The listing builds one solid part. Answer for the finished solid, in the listing's coordinates (mm). Face numbers are marked on the shaded views. A direction names the side the tool comes from. Give positions to 0.01 mm unless a question says otherwise; leave off trailing zeros. Order: outer loops, then holes, each group sorted by start corner. A loop starts at its lowest first (then second) coordinate and runs counter-clockwise, first axis right, second up. Notation, with made-up numbers: (76.25, 30) - (123.25, 30) arc R18 cw to (123.25, 42) - close; hole circle Ø3 at (-30.75, -34). An arc over 180 degrees is marked (long way). Answer as CSV lines item,"result". Start each with the question number.
1. Determine the mould class of the marked faces 1, 2 and 3 for opening direction Y: +Y half, -Y half, draft (parallel to the pull), parting line (faces both ways), or undercut.
2. Which of the six approach directions +Z, -Z, +X, -X, +Y, -Y give full straight-line access (tool end or side, diameter ignored) to the marked faces 4 and 5?
3. Section D-D on x = 19.5 is taken. Give the vertices of the cut face in (y, z).
4. Consider line 1 along Y through (x, z) = (0, 4.5); line 2 along Y through (x, z) = (0, 0.85); line 3 along Z through (x, y) = (-22.5, 13.5). Determine where each line is inside the solid, lowest interval first. Write a range as [from, to].
5. Section C-C on z = 1 is taken. Give the vertices of the cut face in (x, y), and give its area (3 significant figures).
6. Section A-A on y = 0 is taken. Give the vertices of the cut face in (x, z), and give its area (3 significant figures).
7. Flat-ended cylindrical pins translate along their axes: pin 1 (1.5 mm diameter, centred on x = -18, y = 9.5, fed in from +Z); pin 2 (3 mm diameter, centred on x = 8.5, z = 8.5, fed in from +Y); pin 3 (4 mm diameter, centred on x = -10, z = 7.5, fed in from -Y). Find the tip coordinate at first contact, or state that the pin passes through.
from build123d import *

# Parameters (mm, degrees)
F0_R     = 26.75
F1_DEPTH = 2
F2_R     = 13.75
F2_R_2   = 12.25
F3_DEPTH = 9.5
F4_SIZE2 = 2
F4_SIZE  = 0.8
F5_R     = 5.5
F6_DEPTH = 25


# Not quite as in the source:
# - a feature of the source that left no trace in its solid (it failed there, or was rolled back) is left out


with BuildPart() as f1:
    # F0 (on Top) → F1 (new body)
    with BuildSketch(Plane.XY):
        Circle(F0_R)
    extrude(amount=F1_DEPTH)

    # F2 (on face) → F3 (join)
    with BuildSketch(Plane.XY.offset(2)):
        Circle(F2_R)
        Circle(F2_R_2, mode=Mode.SUBTRACT)
    extrude(amount=F3_DEPTH)

    # F4
    f4_edges = [f1.edges().sort_by_distance(p)[0] for p in [
        (-13.75, 0, 11.5),
    ]]
    f4_side = f1.faces().sort_by_distance((-13.361091, 0, 11.5))[0]
    chamfer(f4_edges, length=F4_SIZE, length2=F4_SIZE2, reference=f4_side)

    # F5 (on face) → F6 (cut)
    with BuildSketch(Plane.XY.offset(2)):
        Circle(F5_R)
    extrude(amount=-F6_DEPTH, mode=Mode.SUBTRACT)


solid = f1.part
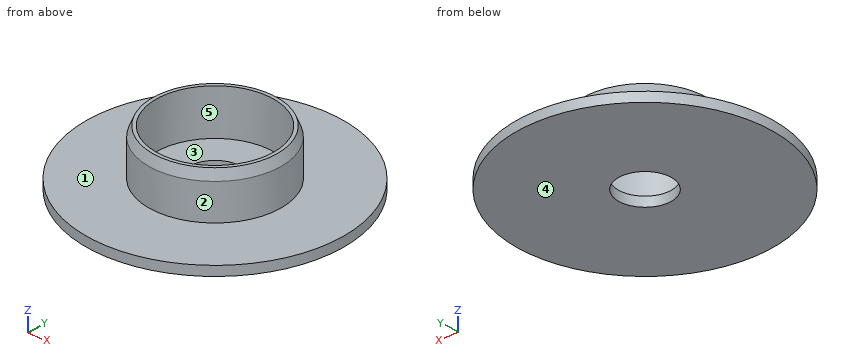
Checks:
1,face 1,"draft"
1,face 2,"parting line"
1,face 3,"undercut"
2,face 4,"-Z, +X, -X, +Y, -Y"
2,face 5,"+Z"
3,outline,"(-18.31, 0) - (18.31, 0) - (18.31, 2) - (-18.31, 2) - close"
4,line 1,"y = [-13.75, -12.25], [12.25, 13.75]"
4,line 2,"y = [-26.75, -5.5], [5.5, 26.75]"
4,line 3,"z = [0, 2]"
5,outline,"circle Ø53.5 at (0, 0); hole circle Ø11 at (0, 0)"
5,area,"2,150 mm²"
6,outline,"(-26.75, 0) - (-5.5, 0) - (-5.5, 2) - (-12.25, 2) - (-12.25, 11.5) - (-12.95, 11.5) - (-13.75, 9.5) - (-13.75, 2) - (-26.75, 2) - close; (5.5, 0) - (26.75, 0) - (26.75, 2) - (13.75, 2) - (13.75, 9.5) - (12.95, 11.5) - (12.25, 11.5) - (12.25, 2) - (5.5, 2) - close"
6,area,"112 mm²"
7,pin 1,"stops at z = 2"
7,pin 2,"stops at y = 11.83"
7,pin 3,"stops at y = -11.18"
